For this review, take the finished solid that the model builds, in its own axes (mm). Face numbers are marked on the shaded views. A direction names the side the tool comes from. Coordinates: 2 decimals unless noted, no trailing zeros. Order: outer loops, then holes, each group sorted by start corner. A loop starts at its lowest first (then second) coordinate and runs counter-clockwise, first axis right, second up.
from build123d import *

# Parameters (mm, degrees)
EXTRUDE_1_DEPTH        = 40
HOLE_WIZARD_M4_1_D     = 3.3
HOLE_WIZARD_M4_1_DEPTH = 10.1
HOLE_WIZARD_M4_1_TIP   = 0.991420021
HOLE_WIZARD_M4_2_D     = 3.3
HOLE_WIZARD_M4_2_DEPTH = 10.1
HOLE_WIZARD_M4_2_TIP   = 0.991420021


with BuildPart() as part:
    # 草图1 → 凸台-拉伸1 (new body)
    with BuildSketch(Plane(origin=(0, 0, 0), x_dir=(1, 0, 0), z_dir=(0, 1, 0))):
        Polygon((0, 0), (20, 0), (10, 17.320508076), align=None)
    extrude(amount=EXTRUDE_1_DEPTH)

    # M4 螺纹孔1
    with Locations(Plane(origin=(0, 0, 0), x_dir=(-1, 0, 0), z_dir=(0, -1, 0))):
        with Locations((-10, 7.320508076)):
            Hole(HOLE_WIZARD_M4_1_D / 2, depth=HOLE_WIZARD_M4_1_DEPTH)
            with Locations((0, 0, -(HOLE_WIZARD_M4_1_DEPTH + HOLE_WIZARD_M4_1_TIP / 2))):  # 118° drill point
                Cone(0, HOLE_WIZARD_M4_1_D / 2, HOLE_WIZARD_M4_1_TIP, mode=Mode.SUBTRACT)

    # M4 螺纹孔2
    with Locations(Plane(origin=(0, 40, 0), x_dir=(1, 0, 0), z_dir=(0, 1, 0))):
        with Locations((10, 7.320508076)):
            Hole(HOLE_WIZARD_M4_2_D / 2, depth=HOLE_WIZARD_M4_2_DEPTH)
            with Locations((0, 0, -(HOLE_WIZARD_M4_2_DEPTH + HOLE_WIZARD_M4_2_TIP / 2))):  # 118° drill point
                Cone(0, HOLE_WIZARD_M4_2_D / 2, HOLE_WIZARD_M4_2_TIP, mode=Mode.SUBTRACT)


solid = part.part
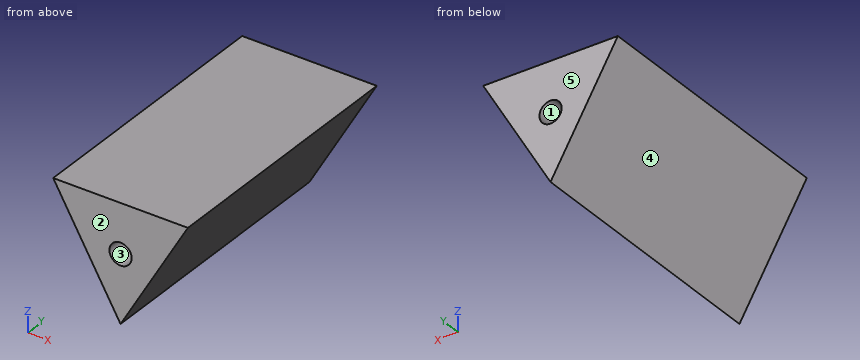
1. Take a section at C-C, the plane y = 16. Give the boundary of the cut face in (x, z).
Answer below:
outline: (0, 0) - (10, -17.32) - (20, 0) - close
2. To check wall thickness, follow L1, parallel to X at y = 11, z = -7.25; L2, parallel to X at y = 33, z = -8; L3, parallel to Z at x = 9, y = 34. State the ranges of each line that lie inside material, in increasing order.
Answer below:
L1: x = 4.19 to 9.87, 10.13 to 15.81
L2: x = 4.62 to 8.5, 11.5 to 15.38
L3: z = -15.59 to -8.63, -6.01 to 0
3. Machinability: for the marked faces 1 and 2, which of the approach directions +Z, -Z, +X, -X, +Y, -Y give a long, thin tool a straight path to every point of the face, cutting with its end or side? Answer none if there is none.
Answer below:
face 1: +Y
face 2: +Z, -Z, +X, -X, -Y
4. Clearance check with flat-ended pins moving along their axes: pin 1 Ø1 at (y, z) = (24, -13) entering from -X; pin 2 Ø2.5 at (x, z) = (10, -7.32) entering from +Y; pin 3 Ø1 at (y, z) = (4, -2) entering from -X. State where each tip first meets the part, or that it passes through.
Answer below:
pin 1: stops at x = 7.22
pin 2: stops at y = 29.66
pin 3: stops at x = 0.87
5. Take a section at B-B, the plane z = -4.75. Give the boundary of the cut face in (x, y), plus the area to 3 significant figures.
Answer below:
outline: (2.74, 0) - (17.26, 0) - (17.26, 40) - (2.74, 40) - close
area: 581 mm2
6. The part is to be moulded in two halves that separate along X. For the marked faces 3, 4 and 5, say which applies: +X half, -X half, draft (parallel to the pull), parting line (faces both ways), or undercut.
Answer below:
face 3: undercut
face 4: -X half
face 5: draft
7. Take a section at D-D, the plane x = 2. Give the boundary of the cut face in (y, z), plus the area to 3 significant figures.
Answer below:
outline: (0, -3.46) - (40, -3.46) - (40, 0) - (0, 0) - close
area: 139 mm2
8. Take a section at A-A, the plane y = 4. Give the boundary of the cut face in (x, z).
Answer below:
outline: (0, 0) - (10, -17.32) - (20, 0) - close; hole circle Ø3.3 at (10, -7.32)
